Geometry: final body of the model. Coordinates: model frame, mm. Face numbers are marked on the shaded views. Coordinates: 2 decimals unless noted, no trailing zeros. Write each loop counter-clockwise with the first axis right and the second up, starting at its lowest first coordinate (ties: lowest second). Pieces come first, ordered by that corner, then holes. Notation, with made-up numbers: (76.5, 7) -> (124.5, 7) arc R20 ccw to (124.5, 45) -> close; hole circle Ø8 at (21, -23). An arc over 180 degrees is marked (long way). One line per item, written item: value.
Autodesk Inventor part; units mm, degrees
ref_plane "YZ Plane" through (0, 0, 0) normal (1, 0, 0) x (0, 1, 0)
ref_plane "XZ Plane" through (0, 0, 0) normal (0, 1, 0) x (-1, 0, 0)
ref_plane "XY Plane" through (0, 0, 0) normal (0, 0, 1) x (1, 0, 0)
sketch "Sketch1" plane through (0, 0, 0) normal (0, 1, 0) x (-1, 0, 0)
  line L0 (-50, 45) -> (-50, -45)
  line L1 (-45, -50) -> (45, -50)
  line L2 (50, -45) -> (50, 45)
  line L3 (45, 50) -> (-45, 50)
  circle A0 centre (46.4645, 46.4645) radius 2
  arc A1 (50, 45) -> (45, 50) centre (45, 45) ccw
  circle A2 centre (45.0503, -45.0503) radius 2
  arc A3 (45, -50) -> (50, -45) centre (45, -45) ccw
  line L4 (48.5355, -48.5355) -> (50, -50) construction
  circle A4 centre (-46.4645, 46.4645) radius 2
  circle A5 centre (-46.4645, -46.4645) radius 2
  arc A6 (-45, 50) -> (-50, 45) centre (-45, 45) ccw
  arc A7 (-50, -45) -> (-45, -50) centre (-45, -45) ccw
  line L5 (-50, 50) -> (-47.8787, 47.8787) construction
  line L6 (-45.0503, 45.0503) -> (46.4645, -46.4645) construction
  line L7 (-50, -50) -> (-47.8787, -47.8787) construction
  line L8 (-45.0503, -45.0503) -> (45.0503, 45.0503) construction
  point P0 (0, 0)
  dimension "d0" = 100
  dimension "d1" = 100
extrude "Extrusion1" add sketch "Sketch1" along normal blind 50
sketch "Sketch2" plane through (0, 50, 0) normal (0, 1, 0) x (1, 0, 0)
  circle A0 centre (0, 0) radius 25
extrude "Extrusion2" add sketch "Sketch2" along normal blind 50
sketch "Sketch3" plane through (0, 100, 0) normal (0, 1, 0) x (1, 0, 0)
  circle A0 centre (0, 0) radius 20
  dimension "d18" = 40
extrude "Extrusion3" cut sketch "Sketch3" against normal blind 30
thread "Thread1"
fillet "Fillet1" radius 2 1 edges at (-25, 100, 0)
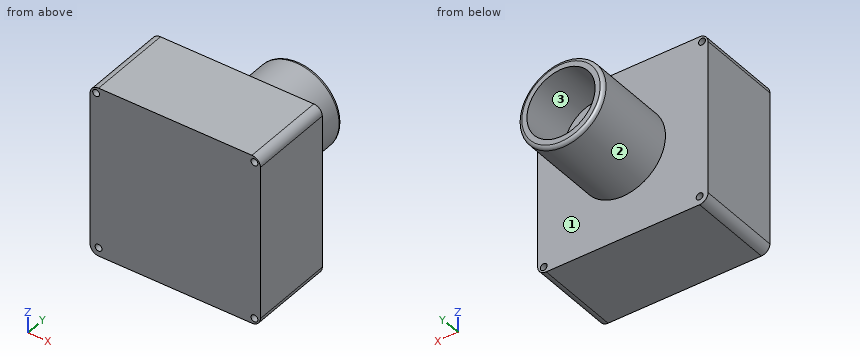
(1) Line query: line 1 (Y direction, x = 13, z = 8); line 2 (Z direction, x = 0.5, y = 80.5) (3 decimals); line 3 (Y direction, x = 34, z = 14.5). Output: solid intervals per line, ascending. Write a range as [from, to].
Responses:
line 1: y = [0, 70]
line 2: z = [-24.995, -19.994], [19.994, 24.995]
line 3: y = [0, 50]
(2) Section C-C (z = -33). Return the cut outline in (x, y).
Responses:
outline: (-50, 0) -> (50, 0) -> (50, 50) -> (-50, 50) -> close
(3) Section A-A (z = 0). Return the cut outline in (x, y), then the cut area to 3 significant figures.
Responses:
outline: (-50, 0) -> (50, 0) -> (50, 50) -> (25, 50) -> (25, 98) arc R2 ccw to (23, 100) -> (20, 100) -> (20, 70) -> (-20, 70) -> (-20, 100) -> (-23, 100) arc R2 ccw to (-25, 98) -> (-25, 50) -> (-50, 50) -> close
area: 6,300 mm2
(4) Pull-direction query (Z, two-part tool) for the marked faces 1, 2 and 3; classes: released by +Z, released by -Z, zero draft, split by the parting line, or undercut.
Responses:
face 1: zero draft
face 2: split by the parting line
face 3: undercut
(5) First-contact query: pin 1 (5 mm diameter, centred on x = -28, z = 20.5, fed in from -Y); pin 2 (1 mm diameter, centred on y = 83, z = 14, fed in from -X); pin 3 (5 mm diameter, centred on x = 46.46, z = -46.46, fed in from +Y); pin 4 (2.5 mm diameter, centred on x = -46.46, z = 46.46, fed in from +Y). Flat tips, straight axial feed; report the tip coordinate or a pass-through.
Responses:
pin 1: stops at y = 0
pin 2: stops at x = -21.04
pin 3: stops at y = 50
pin 4: passes through
(6) Section D-D (x = -36). Return the cut outline in (y, z).
Responses:
outline: (0, -50) -> (50, -50) -> (50, 50) -> (0, 50) -> close
(7) Section B-B (x = 0). Return the cut outline in (y, z), then the cut area to 3 significant figures.
Responses:
outline: (0, -50) -> (50, -50) -> (50, -25) -> (98, -25) arc R2 ccw to (100, -23) -> (100, -20) -> (70, -20) -> (70, 20) -> (100, 20) -> (100, 23) arc R2 ccw to (98, 25) -> (50, 25) -> (50, 50) -> (0, 50) -> close
area: 6,300 mm2
